Build history of the part. All positions in model axes, mm. A direction names the side the tool comes from. Round coordinates to 2 decimals unless told otherwise and drop trailing zeros. Write each loop counter-clockwise with the first axis right and the second up, starting at its lowest first coordinate (ties: lowest second). Pieces come first, ordered by that corner, then holes. Notation, with made-up numbers: (89.25, 62.5) -> (105.25, 62.5) arc R21 cw to (105.25, 84.5) -> close; hole circle Ø10 at (44, -11.75). An arc over 180 degrees is marked (long way). Answer in a Markdown table with one row per item.
```python
from build123d import *

# Parameters (mm, degrees)
ESTRUSIONE_ESTRUSIONE1_DEPTH                         = 6
SCHIZZO3_W                                           = 136.2
SCHIZZO3_H                                           = 72.5
ESTRUSIONE_ESTRUSIONE2_DEPTH                         = 6
TAGLIO_ESTRUSIONE1_DEPTH                             = 131.797324132
RACCORDO5_R                                          = 15
ESTRUSIONE_ESTRUSIONE5_DEPTH                         = 6
ESTRUSIONE_ESTRUSIONE5_DEPTH_BACK                    = 60
SCHIZZO9_W                                           = 6
SCHIZZO9_H                                           = 33.15279029
RACCORDO6_R                                          = 5
RACCORDO7_R                                          = 5
FORO_LAMATO_PER_BULLONE_M3_A_TESTA_E_2_COUNT         = 2
FORO_LAMATO_PER_BULLONE_M3_A_TESTA_E_2_PITCH         = 10.95
FORO_LAMATO_PER_BULLONE_M5_A_TESTA_ESAGO_D           = 5.5
FORO_LAMATO_PER_BULLONE_M5_A_TESTA_ESAGO_CBORE_D     = 12.238
FORO_LAMATO_PER_BULLONE_M5_A_TESTA_ESAGO_CBORE_DEPTH = 3.5


with BuildPart() as part:
    # Schizzo2 → Estrusione-Estrusione1 (new body)
    with BuildSketch(Plane.XY):
        with BuildLine():
            Line((-27.5, 0), (-27.5, 45))
            ThreePointArc((-27.5, 45), (0, 72.5), (27.5, 45))
            Line((27.5, 45), (27.5, 0))
            ThreePointArc((27.5, 0), (0, -27.5), (-27.5, 0))
        make_face()
    extrude(amount=ESTRUSIONE_ESTRUSIONE1_DEPTH)

    # Schizzo3 → Estrusione-Estrusione2 (add)
    with BuildSketch(Plane.XY):
        with Locations((-40.6, 36.25)):
            Rectangle(SCHIZZO3_W, SCHIZZO3_H)
    extrude(amount=ESTRUSIONE_ESTRUSIONE2_DEPTH)

    # Schizzo4 → Taglio-Estrusione1 (cut, through all)
    with BuildSketch(Plane.XY.offset(6)):
        Polygon((-27.5, 0), (-108.7, 0), (-108.7, 39.34720971), (-27.5, 14.142426235), align=None)
    extrude(amount=-TAGLIO_ESTRUSIONE1_DEPTH, mode=Mode.SUBTRACT)

    # Raccordo5
    raccordo5_edges = [part.edges().sort_by_distance(p)[0] for p in [
        (-27.5, 14.142426235, 3),
    ]]
    fillet(raccordo5_edges, radius=RACCORDO5_R)

    # Schizzo9 → Estrusione-Estrusione5 (add, two sides: drawn at the far end of the back side and taken through both)
    with BuildSketch(Plane.XY.offset(-ESTRUSIONE_ESTRUSIONE5_DEPTH_BACK)):
        with Locations((-111.7, 55.923604855)):
            Rectangle(SCHIZZO9_W, SCHIZZO9_H)
    extrude(amount=ESTRUSIONE_ESTRUSIONE5_DEPTH + ESTRUSIONE_ESTRUSIONE5_DEPTH_BACK)

    # Raccordo6
    raccordo6_edges = [part.edges().sort_by_distance(p)[0] for p in [
        (-108.7, 55.923604855, 0),
    ]]
    fillet(raccordo6_edges, radius=RACCORDO6_R)

    # Raccordo7
    raccordo7_edges = [part.edges().sort_by_distance(p)[0] for p in [
        (-114.7, 55.923604855, 6),
    ]]
    fillet(raccordo7_edges, radius=RACCORDO7_R)

    # Schizzo20 → Foro lamato per Bullone M3 a testa esagonale-3 (revolve, cut)
    with BuildSketch(Plane(origin=(0, 67, 0), x_dir=(0, 1, 0), z_dir=(1, 0, 0))):
        Polygon((0, 0), (0, 6), (1.7, 6), (1.7, 0.5), (4.5, 0.5), (4.5, 0.025), (4.525, 0), align=None)
    foro_lamato_per_bullone_m3_a_testa_esago = revolve(axis=Axis((0, 67, -6.35), (0, 0, 1)), mode=Mode.SUBTRACT)

    # Foro lamato per Bullone M3 a testa e 2: Foro lamato per Bullone M3 a testa esagonale-3 ×2
    with Locations(*[(0, -i * FORO_LAMATO_PER_BULLONE_M3_A_TESTA_E_2_PITCH, 0) for i in range(1, FORO_LAMATO_PER_BULLONE_M3_A_TESTA_E_2_COUNT)]):
        add(foro_lamato_per_bullone_m3_a_testa_esago, mode=Mode.SUBTRACT)

    # Foro lamato per Bullone M5 a testa esagonale-1 (through all)
    with Locations(Plane.XY.offset(6)):
        with Locations((0, 0)):
            CounterBoreHole(FORO_LAMATO_PER_BULLONE_M5_A_TESTA_ESAGO_D / 2, FORO_LAMATO_PER_BULLONE_M5_A_TESTA_ESAGO_CBORE_D / 2, FORO_LAMATO_PER_BULLONE_M5_A_TESTA_ESAGO_CBORE_DEPTH)


solid = part.part
```
Q1. Drop flat-ended pins along their axis: P1, Ø1.8, axis at x = -111, z = -23.5, coming from the -Y side; P2, Ø7, axis at x = -2, y = 67, coming from the -Z side; P3, Ø10, axis at x = 0, y = 0, coming from the +Z side. Give the stop position or say it passes through.
A:
| item | result |
|---|---|
| P1 | y = 39.35 |
| P2 | z = 0 |
| P3 | z = 2.5 |
Q2. Wall check: line 1 (Y direction, x = 0, z = 4); line 2 (Y direction, x = 0, z = 2.15); line 3 (X direction, y = 56.05, z = 0.2). Give the ranges that are in metal, low to high. Write a range as [from, to].
A:
| item | result |
|---|---|
| line 1 | [-27.5, -6.12], [6.12, 54.35], [57.75, 65.3], [68.7, 72.5] |
| line 2 | [-27.5, -2.75], [2.75, 54.35], [57.75, 65.3], [68.7, 72.5] |
| line 3 | [-114.7, -4.5], [4.5, 27.5] |
Q3. Saw through at A-A on x = 0. State how many separate pieces and enclosed holes the cut face has, plus the area to 3 significant figures.
A:
| item | result |
|---|---|
| separate pieces | 4 |
| enclosed holes | 0 |
| area | 497 mm² |
Q4. Two-plate mould, pull along Y, no slides. Class faces 4 (the flat face through (-65, 72.5, 2)), 5 (the flat face through (-27, 34, 6)), 6 (the cylindrical face through (-1.326, -5.973, 4.274)): released by +Y, released by -Y, zero draft, split by the parting line, or undercut.
A:
| item | result |
|---|---|
| face 4 | released by +Y |
| face 5 | zero draft |
| face 6 | undercut |
Q5. Which spindle directions (+Z, -Z, +X, -X, +Y, -Y) get a long thin tool onto all of the face, cutting with end or side? Do faces 1 (the flat face through (-24, 34, 0)), 2 (the flat face through (1, -3, 2.5)), 3 (the flat face through (-27.5, 2, 3)). Say none if no direction does.
A:
| item | result |
|---|---|
| face 1 | -Z, +X, +Y, -Y |
| face 2 | +Z |
| face 3 | +Z, -Z, -X, -Y |
Q6. Saw through at C-C on z = -36.5. Write the cut outline in (x, y).
A:
| item | result |
|---|---|
| outline | (-114.7, 39.35) -> (-108.7, 39.35) -> (-108.7, 72.5) -> (-114.7, 72.5) -> close |
Q7. Saw through at D-D on y = 29. Write the cut outline in (x, z), plus the area to 3 significant figures.
A:
| item | result |
|---|---|
| outline | (-75.37, 0) -> (27.5, 0) -> (27.5, 6) -> (-75.37, 6) -> close |
| area | 617 mm² |
Q8. Saw through at B-B on y = 67. Write the cut outline in (x, z) (3 decimals).
A:
| item | result |
|---|---|
| outline | (-114.7, -60) -> (-108.7, -60) -> (-108.7, -5) arc R5 cw to (-103.7, 0) -> (-4.525, 0) -> (-4.5, 0.025) -> (-4.5, 0.5) -> (-1.7, 0.5) -> (-1.7, 6) -> (-109.7, 6) arc R5 ccw to (-114.7, 1) -> close; (1.7, 0.5) -> (4.5, 0.5) -> (4.5, 0.025) -> (4.525, 0) -> (27.5, 0) -> (27.5, 6) -> (1.7, 6) -> close |
